Source: CAD feature listing. Evaluate the final solid. Frame: model axes, mm. A direction names the side the tool comes from. Round coordinates to 2 decimals unless told otherwise and drop trailing zeros. Loops run counter-clockwise (first coordinate to the right, second up) from the corner with the lowest first, then second, coordinate; pieces in that order, holes last.
Item 1: First-contact query: P1, Ø8, axis at x = 3.5, z = -7.5, coming from the -Y side; P2, Ø4, axis at y = 55, z = 3, coming from the +X side; P3, Ø12, axis at y = 57, z = 11.5, coming from the -X side; P4, Ø3, axis at x = -1, z = 13.5, coming from the +Y side. Flat tips, straight axial feed; report the tip coordinate or a pass-through.
Item 2: Section query B-B on y = 28. Return loops of the section in (x, z), then the cut area to 3 significant figures.
Item 3: Pull-direction query (X, two-part tool) for faces 4 (the cylindrical face through (-10.74, 103.49, -2.38)), 5 (the flat face through (14, 97.5, 0)), 6 (the flat face through (0, 97.5, 14)), 7 (the flat face through (-5, 104.5, 0)); classes: released by +X, released by -X, zero draft, split by the parting line, or undercut.
Item 4: Ray query, L1, parallel to X at y = 101.2, z = 0; L2, parallel to X at y = 99.5, z = -1; L3, parallel to Y at x = 10, z = -5.5. Return the intervals inside material, ascending.
Item 5: Access query for faces 1 (the flat face through (0, 0, 0)), 2 (the flat face through (0, 117, -2.426)), 3 (the cylindrical face through (-1.2, 100, 12.4)). Directions: +Z, -Z, +X, -X, +Y, -Y. A direction counts if a zero-diameter tool reaches every point of the face in a straight line with its end or side. Return the directions, or none.
```python
from build123d import *

# Parameters (mm, degrees)
SKETCH_1_R          = 18
EXTRUDE_1_DEPTH     = 60
FILLET_1_R          = 1
SKETCH_3_R          = 18
EXTRUDE_2_DEPTH     = 42.5
SKETCH_4_R          = 11
EXTRUDE_3_DEPTH     = 2
SKETCH_5_R          = 4
EXTRUDE_4_DEPTH     = 20
CUT_EXTRUDE_START   = -15
CUT_EXTRUDE_1_DEPTH = 15
SKETCH_7_R          = 2
CUT_EXTRUDE_2_DEPTH = 5


with BuildPart() as part:
    # 草图1 → 凸台-拉伸1 (new body)
    with BuildSketch(Plane(origin=(0, 0, 0), x_dir=(1, 0, 0), z_dir=(0, 1, 0))):
        with Locations(Location((0, 0, 0), (0, 0, 270))):
            Circle(SKETCH_1_R)
    extrude(amount=EXTRUDE_1_DEPTH)

    # 圆角1
    fillet_1_edges = [part.edges().sort_by_distance(p)[0] for p in [
        (0, 0, -18),
        (0, 60, -18),
    ]]
    fillet(fillet_1_edges, radius=FILLET_1_R)

    # 草图3 → 凸台-拉伸2 (add)
    with BuildSketch(Plane(origin=(0, 60, 0), x_dir=(1, 0, 0), z_dir=(0, 1, 0))):
        with Locations(Location((0, 0, 0), (0, 0, 270))):
            Circle(SKETCH_3_R)
    extrude(amount=EXTRUDE_2_DEPTH)

    # 草图4 → 凸台-拉伸3 (add)
    with BuildSketch(Plane(origin=(0, 102.5, 0), x_dir=(1, 0, 0), z_dir=(0, 1, 0))):
        with Locations(Location((0, 0, 0), (0, 0, 270))):
            Circle(SKETCH_4_R)
    extrude(amount=EXTRUDE_3_DEPTH)

    # 草图5 → 凸台-拉伸4 (add)
    with BuildSketch(Plane(origin=(0, 104.5, 0), x_dir=(1, 0, 0), z_dir=(0, 1, 0))):
        with Locations(Location((0, 0, 0), (0, 0, 270))):
            Circle(SKETCH_5_R)
    extrude(amount=EXTRUDE_4_DEPTH)

    # 草图6 → 切除-拉伸1 (cut)
    with BuildSketch(Plane(origin=(0, 124.5, 0), x_dir=(1, 0, 0), z_dir=(0, 1, 0)).offset(CUT_EXTRUDE_START)):
        with BuildLine():
            Line((-3.180068641, 2.426347758), (3.180068641, 2.426347758))
            ThreePointArc((3.180068641, 2.426347758), (0, 4), (-3.180068641, 2.426347758))
        make_face()
    extrude(amount=CUT_EXTRUDE_1_DEPTH, mode=Mode.SUBTRACT)

    # 草图7 → 切除-拉伸2 (cut)
    with BuildSketch(Plane(origin=(0, 102.5, 0), x_dir=(1, 0, 0), z_dir=(0, 1, 0))):
        with Locations(Location((0, 14, 0), (0, 0, 270))):
            Circle(SKETCH_7_R)
        with Locations(Location((14, 0, 0), (0, 0, 270))):
            Circle(SKETCH_7_R)
        with Locations(Location((0, -14, 0), (0, 0, 270))):
            Circle(SKETCH_7_R)
        with Locations(Location((-14, 0, 0), (0, 0, 270))):
            Circle(SKETCH_7_R)
    extrude(amount=-CUT_EXTRUDE_2_DEPTH, mode=Mode.SUBTRACT)


solid = part.part
```
Data:
1. P1: stops at y = 0
1. P2: stops at x = 17.97
1. P3: stops at x = -17.14
1. P4: stops at y = 102.5
2. outline: circle Ø36 at (0, 0)
2. area: 1,020 mm2
3. face 4: split by the parting line
3. face 5: undercut
3. face 6: undercut
3. face 7: zero draft
4. L1: x = -18 to -16, -12 to 12, 16 to 18
4. L2: x = -17.97 to -15.73, -12.27 to 12.27, 15.73 to 17.97
4. L3: y = 0 to 102.5
5. face 1: +Z, -Z, +X, -X, -Y
5. face 2: -Z, +X, -X, +Y
5. face 3: +Y
